CAD build for the part. Positions are in the model's coordinates, mm. A direction names the side the tool comes from. Give positions to 0.01 mm unless a question says otherwise; leave off trailing zeros. Loops run counter-clockwise (first coordinate to the right, second up) from the corner with the lowest first, then second, coordinate; pieces in that order, holes last. Notation, with made-up numbers: (-7.75, 46) - (-1.75, 46) arc R26 cw to (-1.75, 73) - close; hole circle Ø9 at (60, -6.5). An arc over 180 degrees is marked (long way). Return JSON: item names as keys, results as strings.
from build123d import *

# Parameters (mm, degrees)
PAD_DEPTH    = 7.5
PAD001_DEPTH = 2.4
FILLET_R     = 5
POCKET_DEPTH = 103.141808
CHAMFER_SIZE = 1


with BuildPart() as part:
    # Sketch → Pad (new body, symmetric)
    with BuildSketch(Plane.XY):
        with BuildLine():
            Line((0, 0), (0, -19))
            ThreePointArc((19, 0), (5.564971, -5.564971), (0, -19))
            Line((19, 0), (0, 0))
        make_face()
    extrude(amount=PAD_DEPTH, both=True)

    # Sketch001 → Pad001 (join, symmetric)
    with BuildSketch(Plane.XY):
        Polygon((0, 0), (0, -25), (-4, -29), (-4, -4), (4, 4), (29, 4), (25, 0), align=None)
    extrude(amount=PAD001_DEPTH, both=True)

    # Fillet
    fillet_edges = [part.edges().sort_by_distance(p)[0] for p in [
        (0, -25, 0),
        (25, 0, 0),
    ]]
    fillet(fillet_edges, radius=FILLET_R)

    # Sketch002 (on Face8 of Fillet) → Pocket (cut, through all)
    with BuildSketch(Plane.XY.offset(2.4)):
        Polygon((-2, -15), (15, -15), (15, 2), (23, 2), (23, -23), (-2, -23), align=None)
    pocket = extrude(amount=POCKET_DEPTH, mode=Mode.SUBTRACT)

    # Mirrored: Pocket across XY
    add(pocket.mirror(Plane.XY), mode=Mode.SUBTRACT)

    # Chamfer
    chamfer_edges = [part.edges().sort_by_distance(p)[0] for p in [
        (0, 0, 4.95),
        (0, 0, -4.95),
    ]]
    chamfer(chamfer_edges, length=CHAMFER_SIZE)


solid = part.part
1. Which spindle directions (+Z, -Z, +X, -X, +Y, -Y) get a long thin tool onto all of the face, cutting with end or side? Do faces 1 (the face through (0.5, -0.5, -4.9)), 2 (the face through (0, -8, 5)), 3 (the face through (21, 0, 0)). Say none if no direction does.
Values follow:
{"face 1": "-Z, -X, +Y", "face 2": "+Z, -X, +Y, -Y", "face 3": "+Z, -Z, +X, -Y"}
2. Cut at A-A, the plane z = 0. Write the cut outline in (x, y).
Values follow:
{"outline": "(-4, -29) - (-1.46, -26.46) arc R5 ccw to (0, -22.93) - (0, -19) arc R19 cw to (19, 0) - (22.93, 0) arc R5 ccw to (26.46, 1.46) - (29, 4) - (4, 4) - (-4, -4) - close"}
3. Cut at B-B, the plane x = 10. Write the cut outline in (y, z).
Values follow:
{"outline": "(-2.27, -7.5) - (0, -7.5) - (0, -2.4) - (4, -2.4) - (4, 2.4) - (0, 2.4) - (0, 7.5) - (-2.27, 7.5) - close"}
4. Cut at D-D, the plane x = 22.5. Write the cut outline in (y, z), plus the area to 3 significant figures.
Values follow:
{"outline": "(0, -2.4) - (4, -2.4) - (4, 2.4) - (0, 2.4) - close", "area": "19.2 mm²"}
5. Drop flat-ended pins along their axis: P1, Ø0.5, axis at x = 0, z = -4.5, coming from the -Y side; P2, Ø1.5, axis at y = -7, z = -5.5, coming from the -X side; P3, Ø4.5, axis at y = -22, z = 0.5, coming from the +X side; P4, Ø1, axis at x = 2.5, y = -14.5, coming from the -Z side. Give the stop position or say it passes through.
Values follow:
{"P1": "stops at y = -15", "P2": "stops at x = 0", "P3": "stops at x = 0", "P4": "passes through"}
6. Cut at C-C, the plane y = -5. Write the cut outline in (x, z), plus the area to 3 significant figures.
Values follow:
{"outline": "(-4, -2.4) - (0, -2.4) - (0, -7.5) - (6.15, -7.5) - (6.15, 7.5) - (0, 7.5) - (0, 2.4) - (-4, 2.4) - close", "area": "112 mm²"}
7. Drill centre lines: probe 1 along Y at (x, z) = (19.5, 1.25); probe 2 along Z at (x, y) = (-1, -9.5); probe 3 along Y at (x, z) = (8.5, -5). Where is each one in solid material? Low to high.
Values follow:
{"probe 1": "y = 0 to 4", "probe 2": "z = -2.4 to 2.4", "probe 3": "y = -3.16 to 0"}
